Input: part model. Units: mm. Frame: model coordinates. Face numbers are marked on the shaded views. A direction names the side the tool comes from. Coordinates: 2 decimals unless noted, no trailing zeros. Write each loop counter-clockwise with the first axis right and the second up, starting at its lowest first coordinate (ties: lowest second). Pieces come first, ordered by that corner, then holes. Notation, with made-up numbers: M 61,12.5 L 116,12.5 A8 cw 116,16.5 Z; hole C 31.25,54.25 d1. An arc over 180 degrees is marked long. Write each question's results on one line, items separated by ' | '. Start each with the question number.
1. First-contact query: pin 1 (11 mm diameter, centred on x = -17.5, y = 10.5, fed in from -Z); pin 2 (1 mm diameter, centred on y = 8.5, z = 88, fed in from -X) (3 decimals); pin 3 (12 mm diameter, centred on y = -20, z = 36, fed in from +X) (3 decimals). Flat tips, straight axial feed; report the tip coordinate or a pass-through.
2. Section query C-C, the plane y = -31. Output: boundary loops of the cut face in (x, z) (3 decimals).
3. Pull-direction query (X, two-part tool) for the marked faces 4, 5, 6 and 7; classes: +X half, -X half, draft (parallel to the pull), parting line (faces both ways), or undercut.
4. Set-up query: the marked faces 1, 2 and 3. Return all of +Z, -Z, +X, -X, +Y, -Y with unobstructed straight access to the full face (end or side cutting, diameter ignored); none if empty.
5. Ray query, probe 1 along X at (y, z) = (-20, 97) (3 decimals); probe 2 along Y at (x, z) = (-35, 15.5); probe 3 along Z at (x, y) = (39, 10). Return the intervals inside material, ascending.
6. Section query B-B, the plane x = 19. Output: boundary loops of the cut face in (y, z).
7. Section query A-A, the plane z = 80.5. Output: boundary loops of the cut face in (x, y) (3 decimals), and give its area (3 significant figures).
8. Section query D-D, the plane x = 47. Output: boundary loops of the cut face in (y, z).
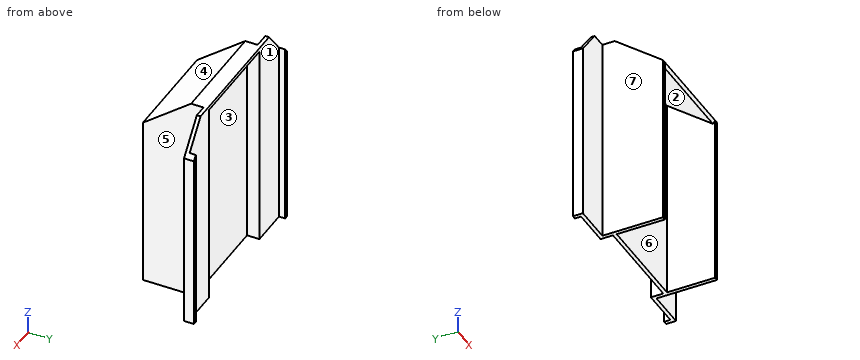
```python
from build123d import *

# Parameters (mm, degrees)
Y_KSEKLIK_EKSTR_ZYON2_DEPTH = 170
KES_EKSTR_ZYON1_DEPTH       = 190.035552212
KES_EKSTR_ZYON1_DEPTH_BACK  = 190.035552212
IZIM3_W                     = 78.85
IZIM3_H                     = 49.045285197
Y_KSEKLIK_EKSTR_ZYON3_DEPTH = 3
KES_EKSTR_ZYON3_DEPTH       = 190.035552212
KES_EKSTR_ZYON3_DEPTH_BACK  = 190.035552212
IZIM5_W                     = 84.85
IZIM5_H                     = 13
Y_KSEKLIK_EKSTR_ZYON4_DEPTH = 3


with BuildPart() as part:
    # Çizim1 → Yükseklik-Ekstrüzyon2 (new body)
    with BuildSketch(Plane.XY):
        Polygon((-39.425, 0), (39.425, 0), (39.425, -38.8), (42.425, -38.8), (42.425, 10), (73, 10), (73, 18), (70, 18), (70, 13), (39.425, 13), (39.425, 3), (-39.425, 3), (-39.425, 13), (-70, 13), (-70, 18), (-73, 18), (-73, 10), (-42.425, 10), (-42.425, -38.8), (-39.425, -38.8), align=None)
    extrude(amount=Y_KSEKLIK_EKSTR_ZYON2_DEPTH)

    # Çizim2 → Kes-Ekstrüzyon1 (cut, two sides: drawn at the far end of the back side and taken through both)
    with BuildSketch(Plane(origin=(0, 0, 0), x_dir=(0, 0, -1), z_dir=(1, 0, 0)).offset(-KES_EKSTR_ZYON1_DEPTH_BACK)):
        Polygon((-170, -38.8), (-170, 0), (-140, -38.8), align=None)
    extrude(amount=KES_EKSTR_ZYON1_DEPTH + KES_EKSTR_ZYON1_DEPTH_BACK, mode=Mode.SUBTRACT)

    # Çizim3 → Yükseklik-Ekstrüzyon3 (add)
    with BuildSketch(Plane(origin=(0, -82.263535985, 106.394173207), x_dir=(1, 0, 0), z_dir=(0, -0.6116795912153945, 0.7911056046385767))):
        with Locations((0, 79.462887909)):
            Rectangle(IZIM3_W, IZIM3_H)
    extrude(amount=-Y_KSEKLIK_EKSTR_ZYON3_DEPTH)

    # Çizim4 → Kes-Ekstrüzyon3 (cut, two sides: drawn at the far end of the back side and taken through both)
    with BuildSketch(Plane(origin=(0, 0, 0), x_dir=(1, 0, 0), z_dir=(0, 1, 0)).offset(-KES_EKSTR_ZYON3_DEPTH_BACK)):
        Polygon((-73, -170), (-73, -146.754135669), (-54.421757633, -170), align=None)
        Polygon((52.86, -170), (73, -170), (73, -144.8), align=None)
    extrude(amount=KES_EKSTR_ZYON3_DEPTH + KES_EKSTR_ZYON3_DEPTH_BACK, mode=Mode.SUBTRACT)

    # Çizim5 → Yükseklik-Ekstrüzyon4 (add)
    with BuildSketch(Plane.XY.offset(170)):
        with Locations((0, 6.5)):
            Rectangle(IZIM5_W, IZIM5_H)
    extrude(amount=-Y_KSEKLIK_EKSTR_ZYON4_DEPTH)


solid = part.part
```
Answer:
1) pin 1: z = 167 | pin 2: x = -42.425 | pin 3: x = 42.425
2) outline: M -42.425,0 L -39.425,0 L -39.425,142.239 L 39.425,142.239 L 39.425,0 L 42.425,0 L 42.425,146.031 L -42.425,146.031 Z
3) face 4: draft | face 5: +X half | face 6: undercut | face 7: -X half
4) face 1: +Z, -Z, +Y | face 2: -Z | face 3: -Z, +Y
5) probe 1: -42.425 to -39.425, 39.425 to 42.425 | probe 2: 0 to 3 | probe 3: 167 to 170
6) outline: M -38.8,140 L -36.96,137.63 L 0,166.21 L 0,0 L 3,0 L 3,167 L 13,167 L 13,170 L 0,170 Z
7) outline: M -73,10 L -42.425,10 L -42.425,-38.8 L -39.425,-38.8 L -39.425,0 L 39.425,0 L 39.425,-38.8 L 42.425,-38.8 L 42.425,10 L 73,10 L 73,18 L 70,18 L 70,13 L 39.425,13 L 39.425,3 L -39.425,3 L -39.425,13 L -70,13 L -70,18 L -73,18 Z | area: 761 mm^2
8) outline: M 10,0 L 13,0 L 13,170 L 10,170 Z
